Source: CAD feature listing. Evaluate the final solid. Frame: model axes, mm. Give positions to 0.01 mm unless a question says otherwise; leave off trailing zeros. Write each loop counter-clockwise with the first axis right and the second up, starting at its lowest first coordinate (ties: lowest second). Pieces come first, ordered by that corner, then holes. Notation, with made-up numbers: M 31,25.5 L 36,25.5 A25 cw 36,38.5 Z; hole C -7,-33.75 d5. An arc over 180 degrees is marked long. Return JSON: item names as keys, results as strings.
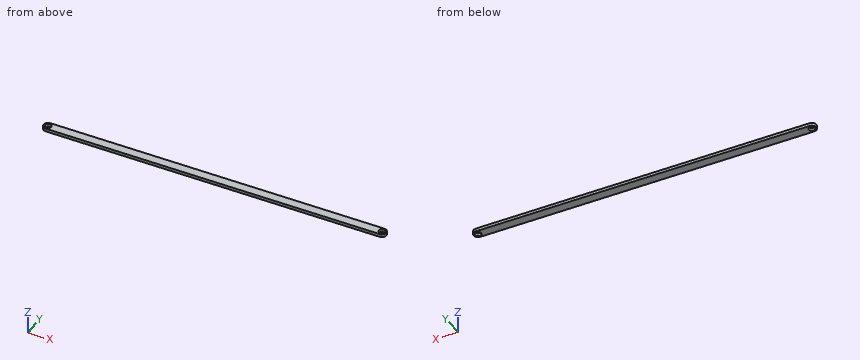
```python
from build123d import *

# Parameters (mm, degrees)
BOSS_EXTRUDE1_DEPTH = 1
CUT_EXTRUDE2_REACH  = 113.515
SKETCH2_R           = 1


with BuildPart() as part:
    # Sketch1 → Boss-Extrude1 (new body)
    with BuildSketch(Plane.XY):
        with BuildLine():
            Line((0, 1.5), (110, 1.5))
            ThreePointArc((110, 1.5), (111.5, 0), (110, -1.5))
            Line((110, -1.5), (0, -1.5))
            ThreePointArc((0, -1.5), (-1.5, 0), (0, 1.5))
        make_face()
    extrude(amount=BOSS_EXTRUDE1_DEPTH)

    # Sketch2 → Cut-Extrude2 (cut, up to next)
    with BuildSketch(Plane.XY.offset(1), mode=Mode.PRIVATE) as cut_extrude2_sk1:
        Circle(SKETCH2_R)
    cut_extrude2_tool1 = extrude(cut_extrude2_sk1.sketch, amount=-CUT_EXTRUDE2_REACH, mode=Mode.PRIVATE) & part.part
    # Sketch2 → Cut-Extrude2 (cut, up to next)
    with BuildSketch(Plane.XY.offset(1), mode=Mode.PRIVATE) as cut_extrude2_sk2:
        with Locations((110, 0)):
            Circle(SKETCH2_R)
    cut_extrude2_tool2 = extrude(cut_extrude2_sk2.sketch, amount=-CUT_EXTRUDE2_REACH, mode=Mode.PRIVATE) & part.part
    add(cut_extrude2_tool1.solids().sort_by_distance((0, 0, 1))[0], mode=Mode.SUBTRACT)
    add(cut_extrude2_tool2.solids().sort_by_distance((110, 0, 1))[0], mode=Mode.SUBTRACT)


solid = part.part
```
1) Cut plane B-B, the plane z = 0.6. Return the cut outline in (x, y).
Numbers:
{"outline": "M 0,-1.5 L 110,-1.5 A1.5 ccw 110,1.5 L 0,1.5 A1.5 ccw Z; hole C 0,0 d2; hole C 110,0 d2"}
2) Contact query for a flat-ended pin moving along its axis: pin 1 Ø1.6 at (x, y) = (0, 0) entering from -Z. Output: stop coordinate, or through.
Numbers:
{"pin 1": "passes through"}
3) Cut plane A-A, the plane y = 0. Return the cut outline in (x, z), then the cut area to 3 significant figures.
Numbers:
{"outline": "M -1.5,0 L -1,0 L -1,1 L -1.5,1 Z; M 1,0 L 109,0 L 109,1 L 1,1 Z; M 111,0 L 111.5,0 L 111.5,1 L 111,1 Z", "area": "109 mm²"}
4) Line query: line 1 (X direction, y = -0.2, z = 0.95); line 2 (Y direction, x = 0, z = 0.65); line 3 (X direction, y = 0.9, z = 0.5). Output: solid intervals per line, ascending. Write a range as [from, to].
Numbers:
{"line 1": "x = [-1.49, -0.98], [0.98, 109.02], [110.98, 111.49]", "line 2": "y = [-1.5, -1], [1, 1.5]", "line 3": "x = [-1.2, -0.44], [0.44, 109.56], [110.44, 111.2]"}
